```python
from build123d import *

# Parameters (mm, degrees)
F1_DEPTH = 63.5
F2_DEPTH = 25.4
F3_DEPTH = 7.9375
F4_R     = 5.08
F5_DEPTH = 12.7


with BuildPart() as f1:
    # F0 (on Front) → F1 (new body, symmetric)
    with BuildSketch(Plane.XZ):
        Polygon((41.275, -22.225), (41.275, 22.225), (28.829001, 22.225), (-41.275, 22.225), (-41.275, -22.225), align=None)
    extrude(amount=F1_DEPTH, both=True)

    # F0 (on Front) → F2 (join, symmetric)
    with BuildSketch(Plane.XZ):
        with BuildLine():
            Line((28.829001, 22.225), (41.275, 22.225))
            Line((41.275, 22.225), (41.275, 36.622151))
            ThreePointArc((41.275, 36.622151), (45.92468, 47.847471), (57.15, 52.497151))
            Line((57.15, 52.497151), (72.650053, 52.497151))
            Line((72.650053, 52.497151), (72.650053, 64.94315))
            Line((72.650053, 64.94315), (57.15, 64.94315))
            ThreePointArc((57.15, 64.94315), (37.124029, 56.648122), (28.829001, 36.622151))
            Line((28.829001, 36.622151), (28.829001, 22.225))
        make_face()
    extrude(amount=F2_DEPTH, both=True)

    # F0 (on Front) → F3 (join, symmetric)
    with BuildSketch(Plane.XZ):
        with BuildLine():
            Line((-41.275, 22.225), (28.829001, 22.225))
            Line((28.829001, 22.225), (28.829001, 36.622151))
            ThreePointArc((28.829001, 36.622151), (37.124029, 56.648122), (57.15, 64.94315))
            add(Edge.make_bspline(
                [(-41.275, 22.225), (-22.058656, 51.323876), (15.271166, 65.268377), (57.15, 64.94315)],
                knots=[0, 0, 0, 0, 107.295484, 107.295484, 107.295484, 107.295484], degree=3))
        make_face()
    extrude(amount=F3_DEPTH, both=True)

    # F4
    f4_edges = [f1.edges().sort_by_distance(p)[0] for p in [
        (41.275, -63.5, 0),
        (-41.275, -63.5, 0),
    ]]
    fillet(f4_edges, radius=F4_R)

    # F0 (on Front) → F5 (join, symmetric)
    with BuildSketch(Plane.XZ):
        Polygon((72.650053, 64.94315), (72.650053, 52.497151), (72.650053, 48.080355), (111.622654, 48.080355), (111.622654, 71.80281), (72.650053, 71.80281), align=None)
    extrude(amount=F5_DEPTH, both=True)


solid = f1.part
```
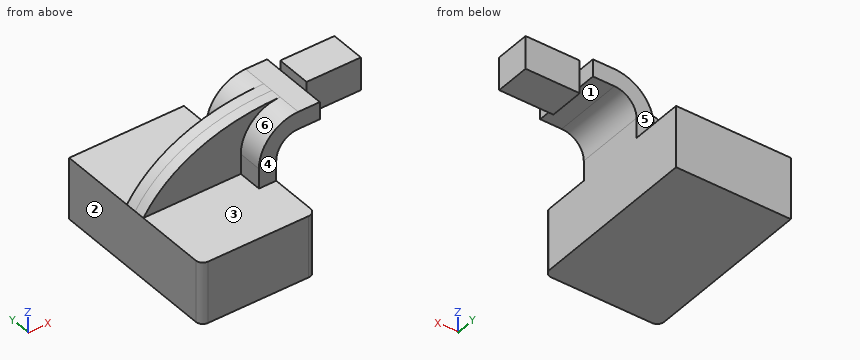
The listing builds one solid part. Answer for the finished solid, in the listing's coordinates (mm). Face numbers are marked on the shaded views. A direction names the side the tool comes from. Give positions to 0.01 mm unless a question says otherwise; leave off trailing zeros. Loops run counter-clockwise (first coordinate to the right, second up) from the corner with the lowest first, then second, coordinate; pieces in that order, holes last. Notation, with made-up numbers: M 49,52 L 71,52 A21 ccw 71,65 Z; hole C 61.5,41.5 d11. An arc over 180 degrees is marked long. One line per item, written item: value.
Q1. A cutting plane is placed at D-D on y = 40.5. Determine the outline of the cut face in (x, z) (3 decimals), then the cut area to 3 significant figures.
Working result:
outline: M -41.275,-22.225 L 41.275,-22.225 L 41.275,22.225 L -41.275,22.225 Z
area: 3,670 mm^2
Q2. A cutting plane is placed at A-A on z = -2. Determine the outline of the cut face in (x, y) (3 decimals).
Working result:
outline: M -41.275,-58.42 A5.08 ccw -36.195,-63.5 L 36.195,-63.5 A5.08 ccw 41.275,-58.42 L 41.275,63.5 L -41.275,63.5 Z
Q3. A cutting plane is placed at B-B on y = 18. Determine the outline of the cut face in (x, z) (3 decimals).
Working result:
outline: M -41.275,-22.225 L 41.275,-22.225 L 41.275,36.622 A15.875 cw 57.15,52.497 L 72.65,52.497 L 72.65,64.943 L 57.15,64.943 A28.321 ccw 28.829,36.622 L 28.829,22.225 L -41.275,22.225 Z
Q4. For the marked faces 4, 5 and 6, determine the directions among +Z, -Z, +X, -X, +Y, -Y from which every point of the face is accessible in a straight line to the end or side of a thin tool.
Working result:
face 4: +Z, +X, -X, -Y
face 5: +Z, +X, -X, +Y
face 6: +Z, -X, -Y
Q5. A cutting plane is placed at C-C on x = 75. Determine the outline of the cut face in (y, z).
Working result:
outline: M -12.7,48.08 L 12.7,48.08 L 12.7,71.8 L -12.7,71.8 Z
Q6. Determine the mould class of the marked faces 1, 2 and 3 for opening direction X: +X half, -X half, draft (parallel to the pull), parting line (faces both ways), or undercut.
Working result:
face 1: undercut
face 2: -X half
face 3: draft
Q7. Find the intervals of material crossed by line 1 (Y direction, x = 35.5, z = 53); line 2 (Z direction, x = 35.5, y = -30) (3 decimals); line 3 (Z direction, x = 103, y = -2.5), in increasing order. Write a range as from..to.
Working result:
line 1: y = -25.4..25.4
line 2: z = -22.225..22.225
line 3: z = 48.08..71.8
Q8. Flat-ended cylindrical pins translate along their axes: P1, Ø17.5, axis at y = -12.5, z = 1.5, coming from the +X side (3 decimals); P2, Ø12, axis at x = 8, z = 51, coming from the +Y side; P3, Ø3, axis at x = -17, y = 24, coming from the +Z side (3 decimals). Find the tip coordinate at first contact, or state that the pin passes through.
Working result:
P1: stops at x = 41.275
P2: stops at y = 7.94
P3: stops at z = 22.225
